Geometry check sheet. Reference: the model listing, model coordinates, mm. A direction names the side the tool comes from. Round coordinates to 2 decimals unless told otherwise and drop trailing zeros. Loops run counter-clockwise (first coordinate to the right, second up) from the corner with the lowest first, then second, coordinate; pieces in that order, holes last. Notation, with made-up numbers: M -7,12.5 L -3,12.5 A18 ccw -3,26.5 Z; hole C -5,72.25 d8. An arc over 180 degrees is marked long. Write item = value, one per line.
from build123d import *

# Parameters (mm, degrees)
F1_DEPTH = 12
F2_R     = 3
F3_DEPTH = 25
F4_R     = 0.75
F5_DEPTH = 6
F6_R     = 2.5
F7_DEPTH = 4


with BuildPart() as f1:
    # F0 (on Front) → F1 (new body)
    with BuildSketch(Plane.XZ):
        Polygon((6.70136, 35.939517), (-38.29864, 35.939517), (-38.29864, 23.939517), (36.70136, 23.939517), (36.70136, 26.439517), align=None)
    extrude(amount=F1_DEPTH)

    # F2 (on face) → F3 (cut)
    with BuildSketch(Plane.XY.offset(35.939517)):
        with Locations((-0.29864, -6)):
            Circle(F2_R)
    extrude(amount=-F3_DEPTH, mode=Mode.SUBTRACT)

    # F4 (on face) → F5 (cut)
    with BuildSketch(Plane.XY.offset(35.939517)):
        with Locations((-8.29864, -6)):
            Circle(F4_R)
    extrude(amount=-F5_DEPTH, mode=Mode.SUBTRACT)

    # F6 (on face) → F7 (cut)
    with BuildSketch(Plane(origin=(0, 0, 23.939517), x_dir=(1, 0, 0), z_dir=(0, 0, -1))):
        with Locations((-30.29864, 6)):
            Circle(F6_R)
    extrude(amount=-F7_DEPTH, mode=Mode.SUBTRACT)


solid = f1.part
(1) Release check for a two-part mould opening along Y. For faces 4 (the flat face through (-10, 0, 30)), 5 (the flat face through (-1, -2, 23.94)), 6 (the flat face through (-30, -6, 27.94)), 7 (the cylindrical face through (-0.689, -3.026, 30.024)) record: released by +Y, released by -Y, zero draft, split by the parting line, or undercut.
Result set:
face_4 = released by +Y
face_5 = zero draft
face_6 = undercut
face_7 = undercut
(2) Depth check by flat-ended pin: pin 1 Ø2.5 at (x, y) = (-29.5, -5.5) entering from -Z; pin 2 Ø2 at (x, y) = (0.5, -7.5) entering from -Z. Enter the tip coordinate at first touch or a pass-through.
Result set:
pin_1 = 27.94
pin_2 = through
(3) Sectioned sample at B-B on z = 25.5. Record the cut outline in (x, y).
Result set:
outline = M -38.3,-12 L 36.7,-12 L 36.7,0 L -38.3,0 Z; hole C -30.3,-6 d5; hole C -0.3,-6 d6
(4) Sectioned sample at D-D on z = 32.25. Record the cut outline in (x, y), then the cut area to 3 significant figures.
Result set:
outline = M -38.3,-12 L 18.35,-12 L 18.35,0 L -38.3,0 Z; hole C -8.3,-6 d1.5; hole C -0.3,-6 d6
area = 650 mm2
(5) Sectioned sample at C-C on y = -11. Record the cut outline in (x, z).
Result set:
outline = M -38.3,23.94 L 36.7,23.94 L 36.7,26.44 L 6.7,35.94 L -38.3,35.94 Z
(6) Material ranges on line 1 along X through (y, z) = (-5, 25.5); line 2 along Y through (x, z) = (-1, 32.5); line 3 along Z through (x, y) = (17, -9), recorded low to high. Write a range as from..to.
Result set:
line_1 = -38.3..-32.59, -28.01..-3.13, 2.53..36.7
line_2 = -12..-8.92, -3.08..0
line_3 = 23.94..32.68
(7) Sectioned sample at A-A on y = -6. Record the cut outline in (x, z).
Result set:
outline = M -38.3,23.94 L -32.8,23.94 L -32.8,27.94 L -27.8,27.94 L -27.8,23.94 L -3.3,23.94 L -3.3,35.94 L -7.55,35.94 L -7.55,29.94 L -9.05,29.94 L -9.05,35.94 L -38.3,35.94 Z; M 2.7,23.94 L 36.7,23.94 L 36.7,26.44 L 6.7,35.94 L 2.7,35.94 Z
(8) Tool access check on faces 1 (the flat face through (-10, -12, 30)), 2 (the cylindrical face through (-32.796, -6.11, 25.912)), 3 (the flat face through (-8, -6, 29.94)). Record the directions out of +Z, -Z, +X, -X, +Y, -Y that give a thin tool (end or side, any length) a straight path to the whole face; none if there is none.
Result set:
face_1 = +Z, -Z, +X, -X, -Y
face_2 = -Z
face_3 = +Z
